```python
from build123d import *

# Parameters (mm, degrees)
SKETCH1_R                = 2.65
SKETCH1_R_2              = 4
SKETCH1_R_3              = 1.8288
SKETCH1_W                = 41.514809608
SKETCH1_H                = 98.81
BOSS_EXTRUDE1_DEPTH      = 3.175
CUT_EXTRUDE1_REACH       = 179.99
SKETCH2_W                = 4.112404804
SKETCH2_H                = 133.245584328
FILLET3_R                = 2.5
FILLET4_R                = 5
M2_5X0_45_TAPPED_HOLE1_D = 2.05


with BuildPart() as part:
    # Sketch1 → Boss-Extrude1 (new body)
    # profile 1 of 8: a face of its own
    with BuildSketch(Plane(origin=(0, 0, 0), x_dir=(0, 0, -1), z_dir=(1, 0, 0))):
        with BuildLine():
            Line((7.5, 134.77502784), (7.5, 117.469314765))
            ThreePointArc((7.5, 117.469314765), (23.361292772, 127.986116465), (29.5, 146))
            ThreePointArc((29.5, 146), (-18.013883535, 169.361292772), (-7.5, 117.469314765))
            Line((-7.5, 117.469314765), (-7.5, 134.77502784))
            ThreePointArc((-7.5, 134.77502784), (-6.363961031, 157.9058809), (13.5, 146))
            ThreePointArc((13.5, 146), (11.9058809, 139.636038969), (7.5, 134.77502784))
        make_face()
        with Locations((-18.619546181, 135.25)):
            Circle(SKETCH1_R, mode=Mode.SUBTRACT)
        with Locations((0, 167.5)):
            Circle(SKETCH1_R, mode=Mode.SUBTRACT)
        with Locations((18.619546181, 135.25)):
            Circle(SKETCH1_R, mode=Mode.SUBTRACT)
    # profile 2 of 8: a face of its own
    with BuildSketch(Plane(origin=(0, 0, 0), x_dir=(0, 0, -1), z_dir=(1, 0, 0))):
        with BuildLine():
            ThreePointArc((-7.5, 117.469314765), (0, 116.5), (7.5, 117.469314765))
            Line((7.5, 117.469314765), (7.5, 134.77502784))
            ThreePointArc((7.5, 134.77502784), (0, 132.5), (-7.5, 134.77502784))
            Line((-7.5, 134.77502784), (-7.5, 117.469314765))
        make_face()
    # profile 3 of 8: a face of its own
    with BuildSketch(Plane(origin=(0, 0, 0), x_dir=(0, 0, -1), z_dir=(1, 0, 0))):
        with BuildLine():
            Line((0, 48.916537522), (6.674602804, 31.57952088))
            ThreePointArc((6.674602804, 31.57952088), (7.290731137, 33.240670729), (7.5, 35))
            Line((7.5, 35), (7.5, 117.469314765))
            ThreePointArc((7.5, 117.469314765), (0, 116.5), (-7.5, 117.469314765))
            Line((-7.5, 117.469314765), (-7.5, 35))
            ThreePointArc((-7.5, 35), (-7.290731137, 33.240670729), (-6.674602804, 31.57952088))
            Line((-6.674602804, 31.57952088), (0, 48.916537522))
        make_face()
    # profile 4 of 8: a face of its own
    with BuildSketch(Plane(origin=(0, 0, 0), x_dir=(0, 0, -1), z_dir=(1, 0, 0))):
        with BuildLine():
            ThreePointArc((-6.674602804, 31.57952088), (0, 27.5), (6.674602804, 31.57952088))
            Line((6.674602804, 31.57952088), (0, 48.916537522))
            Line((0, 48.916537522), (-6.674602804, 31.57952088))
        make_face()
        with Locations((0, 35)):
            Circle(SKETCH1_R_2, mode=Mode.SUBTRACT)
    # profile 5 of 8: a face of its own
    with BuildSketch(Plane(origin=(0, 0, 0), x_dir=(0, 0, -1), z_dir=(1, 0, 0))):
        with BuildLine():
            Line((-20.757404804, -5), (20.757404804, -5))
            Line((20.757404804, -5), (7.5, 29.435584328))
            Line((7.5, 29.435584328), (6.674602804, 31.57952088))
            ThreePointArc((6.674602804, 31.57952088), (0, 27.5), (-6.674602804, 31.57952088))
            Line((-6.674602804, 31.57952088), (-7.5, 29.435584328))
            Line((-7.5, 29.435584328), (-20.757404804, -5))
        make_face()
        with Locations((-13.4747, 0)):
            Circle(SKETCH1_R_3, mode=Mode.SUBTRACT)
        with Locations((13.4747, 0)):
            Circle(SKETCH1_R_3, mode=Mode.SUBTRACT)
    # profile 6 of 8: a face of its own
    with BuildSketch(Plane(origin=(0, 0, 0), x_dir=(0, 0, -1), z_dir=(1, 0, 0))):
        with BuildLine():
            Line((-7.5, 35), (-7.5, 29.435584328))
            Line((-7.5, 29.435584328), (-6.674602804, 31.57952088))
            ThreePointArc((-6.674602804, 31.57952088), (-7.290731137, 33.240670729), (-7.5, 35))
        make_face()
    # profile 7 of 8: a face of its own
    with BuildSketch(Plane(origin=(0, 0, 0), x_dir=(0, 0, -1), z_dir=(1, 0, 0))):
        with BuildLine():
            Line((6.674602804, 31.57952088), (7.5, 29.435584328))
            Line((7.5, 29.435584328), (7.5, 35))
            ThreePointArc((7.5, 35), (7.290731137, 33.240670729), (6.674602804, 31.57952088))
        make_face()
    # profile 8 of 8: a face of its own
    with BuildSketch(Plane(origin=(0, 0, 0), x_dir=(0, 0, -1), z_dir=(1, 0, 0))):
        with Locations((0, -54.405)):
            Rectangle(SKETCH1_W, SKETCH1_H)
        with Locations((13.4747, -100)):
            Circle(SKETCH1_R_3, mode=Mode.SUBTRACT)
        with Locations((-13.4747, -100)):
            Circle(SKETCH1_R_3, mode=Mode.SUBTRACT)
    extrude(amount=BOSS_EXTRUDE1_DEPTH)

    # Sketch2 → Cut-Extrude1 (cut, up to next)
    with BuildSketch(Plane(origin=(3.175, 0, 0), x_dir=(0, 0, -1), z_dir=(1, 0, 0)), mode=Mode.PRIVATE) as cut_extrude1_sk1:
        Polygon((11.645, -5), (-11.645, -5), (11.645, -27.976379872), align=None)
    cut_extrude1_tool1 = extrude(cut_extrude1_sk1.sketch, amount=-CUT_EXTRUDE1_REACH, mode=Mode.PRIVATE) & part.part
    # Sketch2 → Cut-Extrude1 (cut, up to next)
    with BuildSketch(Plane(origin=(3.175, 0, 0), x_dir=(0, 0, -1), z_dir=(1, 0, 0)), mode=Mode.PRIVATE) as cut_extrude1_sk2:
        Polygon((-11.645, -12.023620128), (11.645, -35), (-11.645, -57.976379872), (-11.645, -35), align=None)
    cut_extrude1_tool2 = extrude(cut_extrude1_sk2.sketch, amount=-CUT_EXTRUDE1_REACH, mode=Mode.PRIVATE) & part.part
    # Sketch2 → Cut-Extrude1 (cut, up to next)
    with BuildSketch(Plane(origin=(3.175, 0, 0), x_dir=(0, 0, -1), z_dir=(1, 0, 0)), mode=Mode.PRIVATE) as cut_extrude1_sk3:
        Polygon((-11.645, -72.023620128), (-11.645, -95), (11.645, -95), align=None)
    cut_extrude1_tool3 = extrude(cut_extrude1_sk3.sketch, amount=-CUT_EXTRUDE1_REACH, mode=Mode.PRIVATE) & part.part
    # Sketch2 → Cut-Extrude1 (cut, up to next)
    with BuildSketch(Plane(origin=(3.175, 0, 0), x_dir=(0, 0, -1), z_dir=(1, 0, 0)), mode=Mode.PRIVATE) as cut_extrude1_sk4:
        Polygon((11.645, -42.023620128), (11.645, -65), (11.645, -87.976379872), (-11.645, -65), align=None)
    cut_extrude1_tool4 = extrude(cut_extrude1_sk4.sketch, amount=-CUT_EXTRUDE1_REACH, mode=Mode.PRIVATE) & part.part
    # Sketch2 → Cut-Extrude1 (cut, up to next)
    with BuildSketch(Plane(origin=(3.175, 0, 0), x_dir=(0, 0, -1), z_dir=(1, 0, 0)), mode=Mode.PRIVATE) as cut_extrude1_sk5:
        with Locations((-18.701202402, -37.187207836)):
            Rectangle(SKETCH2_W, SKETCH2_H)
    cut_extrude1_tool5 = extrude(cut_extrude1_sk5.sketch, amount=-CUT_EXTRUDE1_REACH, mode=Mode.PRIVATE) & part.part
    # Sketch2 → Cut-Extrude1 (cut, up to next)
    with BuildSketch(Plane(origin=(3.175, 0, 0), x_dir=(0, 0, -1), z_dir=(1, 0, 0)), mode=Mode.PRIVATE) as cut_extrude1_sk6:
        with Locations((18.701202402, -37.187207836)):
            Rectangle(SKETCH2_W, SKETCH2_H)
    cut_extrude1_tool6 = extrude(cut_extrude1_sk6.sketch, amount=-CUT_EXTRUDE1_REACH, mode=Mode.PRIVATE) & part.part
    add(cut_extrude1_tool1.solids().sort_by_distance((3.175, -12.658793, -3.881667))[0], mode=Mode.SUBTRACT)
    add(cut_extrude1_tool2.solids().sort_by_distance((3.175, -35, 3.881667))[0], mode=Mode.SUBTRACT)
    add(cut_extrude1_tool3.solids().sort_by_distance((3.175, -87.341207, 3.881667))[0], mode=Mode.SUBTRACT)
    add(cut_extrude1_tool4.solids().sort_by_distance((3.175, -65, -3.881667))[0], mode=Mode.SUBTRACT)
    add(cut_extrude1_tool5.solids().sort_by_distance((3.175, -37.187208, 18.701202))[0], mode=Mode.SUBTRACT)
    add(cut_extrude1_tool6.solids().sort_by_distance((3.175, -37.187208, -18.701202))[0], mode=Mode.SUBTRACT)

    # Fillet3
    fillet3_edges = [part.edges().sort_by_distance(p)[0] for p in [
        (1.5875, -72.023620128, 11.645),
        (1.5875, -95, -11.645),
        (1.5875, -95, 11.645),
        (1.5875, -87.976379872, -11.645),
        (1.5875, -65, 11.645),
        (1.5875, -42.023620128, -11.645),
        (1.5875, -27.976379872, -11.645),
        (1.5875, -5, 11.645),
        (1.5875, -5, -11.645),
        (1.5875, -103.81, 16.645),
        (1.5875, -12.023620128, 11.645),
        (1.5875, -35, -11.645),
        (1.5875, -57.976379872, 11.645),
        (1.5875, -103.81, -16.645),
    ]]
    fillet(fillet3_edges, radius=FILLET3_R)

    # Fillet4
    fillet4_edges = [part.edges().sort_by_distance(p)[0] for p in [
        (1.5875, 117.469314765, -7.5),
        (1.5875, 29.435584328, -7.5),
        (1.5875, 29.435584328, 7.5),
        (1.5875, 117.469314765, 7.5),
        (1.5875, 5.681808734, 16.645),
        (1.5875, 5.681808734, -16.645),
    ]]
    fillet(fillet4_edges, radius=FILLET4_R)

    # M2.5x0.45 Tapped Hole1 (through all)
    with Locations(Plane(origin=(3.175, 0, 0), x_dir=(0, 0, -1), z_dir=(1, 0, 0))):
        with Locations((23.015, 146), (-23.015, 146)):
            Hole(M2_5X0_45_TAPPED_HOLE1_D / 2)


solid = part.part
```
Here's how the part is built. I have some questions about the finished solid (model axes, mm). A direction names the side the tool comes from. Round coordinates to 2 decimals unless told otherwise and drop trailing zeros. Order: outer loops, then holes, each group sorted by start corner. A loop starts at its lowest first (then second) coordinate and runs counter-clockwise, first axis right, second up. Notation, with made-up numbers: M 71.25,74.5 L 90.25,74.5 A8 ccw 90.25,87.5 Z; hole C -35,9.25 d4. An arc over 180 degrees is marked long. Answer in a Markdown table with one row per item.
Item 1: Imagine slicing it at B-B, the plane z = 0. State how many separate pieces and enclosed holes the cut face has, and give its area (3 significant figures).
A:
| item | result |
|---|---|
| separate pieces | 8 |
| enclosed holes | 0 |
| area | 540 mm2 |
Item 2: I'm going to push flat-ended pins straight in: pin 1 (1 mm diameter, centred on x = 1, z = 0.5, fed in from +Y); pin 2 (1 mm diameter, centred on x = 2.5, y = -63, fed in from +Z) (3 decimals); pin 3 (1 mm diameter, centred on x = 2, y = -33, fed in from -Z) (3 decimals). Where does each tip first touch, or does it pass through?
A:
| item | result |
|---|---|
| pin 1 | stops at y = 175.5 |
| pin 2 | stops at z = 16.645 |
| pin 3 | stops at z = -16.645 |
Item 3: Thinking about a two-plate mould opening in Z: for faces 1 (the face through (1.565, 132.663, 19.194)), 2 (the face through (0, 69, 0)), 3 (the face through (1.565, 17.713, 12.013)), which applies, +Z half, -Z half, draft (parallel to the pull), parting line (faces both ways), or undercut?
A:
| item | result |
|---|---|
| face 1 | undercut |
| face 2 | draft |
| face 3 | +Z half |
Item 4: For faces 4 (the face through (1.565, 17.405, -12.132)), 5 (the face through (3.175, 69, 0)), 6 (the face through (1.61, -75.398, 1.105)), which set-ups out of +Z, -Z, +X, -X, +Y, -Y let a thin tool reach every point of the face, with its end or its side?
A:
| item | result |
|---|---|
| face 4 | -Z, +X, -X |
| face 5 | +Z, -Z, +X, +Y, -Y |
| face 6 | +X, -X |
Item 5: Imagine slicing it at D-D, the plane y = 70. Write out the boundary of the cut face in (x, z) (3 decimals), and give its area (3 significant figures).
A:
| item | result |
|---|---|
| outline | M 0,-7.5 L 3.175,-7.5 L 3.175,7.5 L 0,7.5 Z |
| area | 47.6 mm2 |
Item 6: If I drill on L1, parallel to Z at x = 1.7, y = -100 (1 decimal); L2, parallel to Z at x = 1.25, y = 135.25; L3, parallel to Y at x = 0.4, z = -6, over which ranges is the centre line in solid material (lowest first)? Write a range as from..to.
A:
| item | result |
|---|---|
| L1 | z = -16.6..-15.3, -11.6..11.6, 15.3..16.6 |
| L2 | z = -27.47..-21.27, -15.97..-8.17, 8.17..15.97, 21.27..27.47 |
| L3 | y = -103.81..-94.96, -89.43..-82.41, -47.59..-40.57, -29.43..-22.41, -5..133.91, 158.09..174.88 |
Item 7: Imagine slicing it at A-A, the plane y = 155.5. Write out the boundary of the cut face in (x, z) (3 decimals).
A:
| item | result |
|---|---|
| outline | M 0,-27.928 L 3.175,-27.928 L 3.175,-9.592 L 0,-9.592 Z; M 0,9.592 L 3.175,9.592 L 3.175,27.928 L 0,27.928 Z |
